```python
from build123d import *

# Parameters (mm, degrees)
SKETCH1_W               = 114.3
SKETCH1_H               = 44.45
BOSS_EXTRUDE1_DEPTH     = 5
BOSS_EXTRUDE2_DEPTH     = 114.3
SKETCH3_R               = 3.025
CUT_EXTRUDE1_DEPTH      = 8
LPATTERN1_COUNT         = 2
LPATTERN1_PITCH         = 38.1
LPATTERN1_COL_COUNT     = 2
LPATTERN1_COL_PITCH     = 38.1
MIRROR1_COPY_1_SKETCH_R = 3.025
MIRROR1_COPY_1_DEPTH    = 8
MIRROR1_COPY_2_SKETCH_R = 3.025
MIRROR1_COPY_2_DEPTH    = 8
SKETCH4_W               = 10.16
SKETCH4_H               = 10.16
BOSS_EXTRUDE3_DEPTH     = 6
M4_CLEARANCE_HOLE1_D    = 4.5
FILLET3_R               = 3.175
FILLET4_R               = 4.7625


with BuildPart() as part:
    # Sketch1 → Boss-Extrude1 (new body)
    with BuildSketch(Plane.XY):
        Rectangle(SKETCH1_W, SKETCH1_H)
    extrude(amount=BOSS_EXTRUDE1_DEPTH)

    # Sketch2 → Boss-Extrude2 (add)
    with BuildSketch(Plane.ZY.offset(57.15)):
        with BuildLine():
            Line((23.8125, 22.225), (5, 22.225))
            Line((5, 22.225), (5, -22.225))
            Line((5, -22.225), (23.8125, -22.225))
            Line((23.8125, -22.225), (23.8125, -12.5269))
            ThreePointArc((23.8125, -12.5269), (11.2856, 0), (23.8125, 12.5269))
            Line((23.8125, 12.5269), (23.8125, 22.225))
        make_face()
    extrude(amount=-BOSS_EXTRUDE2_DEPTH)

    # Sketch3 → Cut-Extrude1 (cut)
    with BuildSketch(Plane.XY.offset(23.8125)):
        with Locations((0, 17.37595)):
            Circle(SKETCH3_R)
    cut_extrude1 = extrude(amount=-CUT_EXTRUDE1_DEPTH, mode=Mode.SUBTRACT)

    # LPattern1: Cut-Extrude1 ×2
    with Locations(*[(i * LPATTERN1_PITCH, 0, 0) for i in range(1, LPATTERN1_COUNT)]):
        add(cut_extrude1, mode=Mode.SUBTRACT)

    # LPattern1 col: Cut-Extrude1 ×2
    with Locations(*[(-i * LPATTERN1_COL_PITCH, 0, 0) for i in range(1, LPATTERN1_COL_COUNT)]):
        add(cut_extrude1, mode=Mode.SUBTRACT)

    # Mirror1: Cut-Extrude1 across plane
    add(cut_extrude1.mirror(Plane.ZX), mode=Mode.SUBTRACT)

    # Mirror1 copy 1 sketch → Mirror1 copy 1 (cut)
    with BuildSketch(Plane(origin=(38.1, 0, 23.8125), x_dir=(1, 0, 0), z_dir=(0, 0, 1))):
        with Locations((0, -17.37595)):
            Circle(MIRROR1_COPY_1_SKETCH_R)
    extrude(amount=-MIRROR1_COPY_1_DEPTH, mode=Mode.SUBTRACT)

    # Mirror1 copy 2 sketch → Mirror1 copy 2 (cut)
    with BuildSketch(Plane(origin=(-38.1, 0, 23.8125), x_dir=(1, 0, 0), z_dir=(0, 0, 1))):
        with Locations((0, -17.37595)):
            Circle(MIRROR1_COPY_2_SKETCH_R)
    extrude(amount=-MIRROR1_COPY_2_DEPTH, mode=Mode.SUBTRACT)

    # Sketch4 → Boss-Extrude3 (add)
    with BuildSketch(Plane.XY):
        Polygon((-65.7225, 30.7975), (-55.5625, 20.6375), (-65.7225, 20.6375), align=None)
        Polygon((-65.7225, 30.7975), (-55.5625, 30.7975), (-55.5625, 20.6375), align=None)
        with Locations((60.6425, -25.7175)):
            Rectangle(SKETCH4_W, SKETCH4_H)
        Polygon((-55.5625, 30.7975), (-60.6425, 25.7175), (-57.15, 22.225), (-55.5625, 22.225), align=None)
        Polygon((-46.99, 22.225), (-55.5625, 30.7975), (-55.5625, 22.225), align=None)
        Polygon((-60.6425, 25.7175), (-65.7225, 20.6375), (-57.15, 20.6375), (-57.15, 22.225), align=None)
        Polygon((-57.15, 20.6375), (-65.7225, 20.6375), (-57.15, 12.065), align=None)
        Polygon((57.15, -20.6375), (65.7225, -20.6375), (57.15, -12.065), align=None)
        Polygon((46.99, -22.225), (55.5625, -30.7975), (55.5625, -22.225), align=None)
    extrude(amount=BOSS_EXTRUDE3_DEPTH)

    # M4 Clearance Hole1 (through all)
    with Locations(Plane.XY.offset(6)):
        with Locations((-60.6425, 25.7175), (60.6425, -25.7175)):
            Hole(M4_CLEARANCE_HOLE1_D / 2)

    # Fillet3
    fillet3_edges = [part.edges().sort_by_distance(p)[0] for p in [
        (-55.5625, 30.7975, 3),
        (-65.7225, 30.7975, 3),
        (-65.7225, 20.6375, 3),
        (55.5625, -30.7975, 3),
        (65.7225, -30.7975, 3),
        (65.7225, -20.6375, 3),
    ]]
    fillet(fillet3_edges, radius=FILLET3_R)

    # Fillet4
    fillet4_edges = [part.edges().sort_by_distance(p)[0] for p in [
        (57.15, -22.225, 14.90625),
        (-57.15, -22.225, 11.90625),
        (-57.15, 22.225, 14.90625),
        (57.15, 22.225, 11.90625),
    ]]
    fillet(fillet4_edges, radius=FILLET4_R)


solid = part.part
```
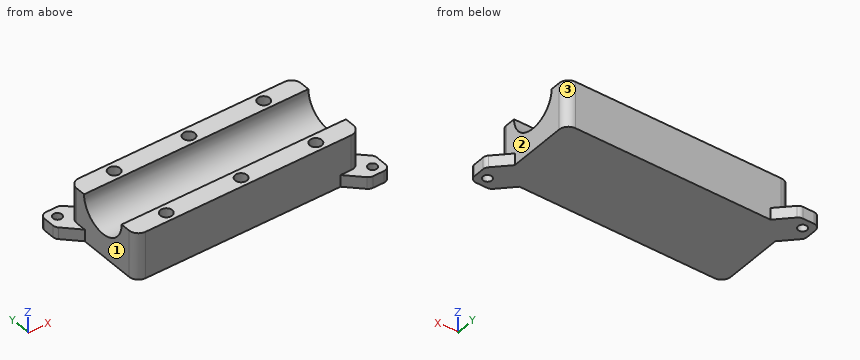
Work out the finished part from the listing and answer in its coordinate system (mm). Face numbers are marked on the shaded views. A direction names the side the tool comes from. Coordinates: 2 decimals unless noted, no trailing zeros. Loops run counter-clockwise (first coordinate to the right, second up) from the corner with the lowest first, then second, coordinate; pieces in that order, holes last.
1) Section D-D (y = 0) is taken. Give the vertices of the cut face in (x, z).
Results:
outline: (-57.15, 0) - (57.15, 0) - (57.15, 11.29) - (-57.15, 11.29) - close
2) For the marked faces 1, 2 and 3, determine the directions among +Z, -Z, +X, -X, +Y, -Y from which every point of the face is accessible in a straight line to the end or side of a thin tool.
Results:
face 1: +Z, -X, -Y
face 2: +Z, +X, +Y
face 3: +Z, -Z, +X, +Y
3) Section A-A (z = 19.5) is taken. Give the number of separate pieces and of enclosed holes in the cut face, plus the area to 3 significant figures.
Results:
separate pieces: 2
enclosed holes: 6
area: 2,200 mm2
4) Section B-B (x = 44.5) is taken. Give the vertices of the cut face in (y, z) (1 decimal), plus the area to 3 significant figures.
Results:
outline: (-22.2, 0) - (22.2, 0) - (22.2, 23.8) - (12.5, 23.8) arc R12.5 cw to (-12.5, 23.8) - (-22.2, 23.8) - close
area: 812 mm2
5) Flat-ended cylindrical pins translate along their axes: pin 1 (3 mm diameter, centred on x = -7, z = 7, fed in from -Y) (3 decimals); pin 2 (3.5 mm diameter, centred on x = 38.1, y = 17.38, fed in from +Z); pin 3 (12 mm diameter, centred on y = 7, z = 15, fed in from +X); pin 4 (8 mm diameter, centred on y = -6, z = 20.5, fed in from -X). Find the tip coordinate at first contact, or state that the pin passes through.
Results:
pin 1: stops at y = -22.225
pin 2: stops at z = 15.81
pin 3: stops at x = 57.15
pin 4: passes through
6) Consider probe 1 along Y at (x, z) = (-38.1, 17.75) (3 decimals); probe 2 along X at (y, z) = (8.5, 2); probe 3 along Z at (x, y) = (58.5, -13.5). Determine where each line is inside the solid, lowest interval first.
Results:
probe 1: y = -22.225 to -20.401, -14.351 to -10.962, 10.962 to 14.351, 20.401 to 22.225
probe 2: x = -57.15 to 57.15
probe 3: z = 0 to 6
